Work out the finished part from the listing and answer in its coordinate system (mm). A direction names the side the tool comes from. Give positions to 0.01 mm unless a question says otherwise; leave off trailing zeros. Order: outer loops, then holes, each group sorted by start corner. A loop starts at its lowest first (then second) coordinate and runs counter-clockwise, first axis right, second up.
```python
from build123d import *

# Parameters (mm, degrees)
F1_DEPTH  = 150
F3_DEPTH  = 15
F3_FACE_R = 12.5031074182
F4_DEPTH  = 15
F4_TAPER  = -45


with BuildPart() as f1:
    # F0 (on Top) → F1 (new body)
    with BuildSketch(Plane.XY):
        Polygon((15.4211589057, 1.0175080366), (3.7976925262, 14.9808209413), (-13.0740558457, 8.2411484845), (-11.8779034096, -9.8875110716), (5.7331078234, -14.3519663908), align=None)
    extrude(amount=F1_DEPTH)

    # F2 (on face) → F3 (join)
    with BuildSketch(Plane.XY.offset(150)):
        with BuildLine():
            ThreePointArc((10.5771332585, -6.6672293454), (12.0119675412, -3.4699179964), (12.5031074182, 0))
            ThreePointArc((12.5031074182, 0), (11.7574524907, 4.2532347737), (9.6094258021, 7.9991643854))
            ThreePointArc((9.6094258021, 7.9991643854), (3.07239751, 12.119738803), (-4.6381823272, 11.6109844463))
            ThreePointArc((-4.6381823272, 11.6109844463), (-10.5771335272, 6.667228919), (-12.4759796348, -0.8231811852))
            ThreePointArc((-12.4759796348, -0.8231811852), (-9.6094258213, -7.9991643624), (-3.0723980071, -12.119738677))
            ThreePointArc((-3.0723980071, -12.119738677), (4.6381814649, -11.6109847907), (10.5771332585, -6.6672293454))
        make_face()
    extrude(amount=F3_DEPTH)

    # F3_face (on face) → F4 (join)
    with BuildSketch(Plane.XY.offset(165)):
        Circle(F3_FACE_R)
    extrude(amount=F4_DEPTH, taper=F4_TAPER)


solid = f1.part
```
1. The part is cut by section B-B (x = 0). Write down the section's boundary in (y, z).
Findings below:
outline: (-27.5, 180) - (-12.5, 165) - (-12.5, 150) - (-12.9, 150) - (-12.9, 0) - (13.46, 0) - (13.46, 150) - (12.5, 150) - (12.5, 165) - (27.5, 180) - close
2. The part is cut by section A-A (z = 60). Write down the section's boundary in (x, y).
Findings below:
outline: (-13.07, 8.24) - (-11.88, -9.89) - (5.73, -14.35) - (15.42, 1.02) - (3.8, 14.98) - close
3. Straight lines are drawn through the part: probe 1 along Z at (x, y) = (-12.5, 3); probe 2 along Z at (x, y) = (-18.5, 3); probe 3 along X at (y, z) = (3, 145). For each, find the intervals that lie inside material, in ascending order.
Findings below:
probe 1: z = 0 to 150, 165.35 to 180
probe 2: z = 171.24 to 180
probe 3: x = -12.73 to 13.77
4. Given P1, Ø5, axis at y = -9.5, z = 149.5, coming from the -X side; P2, Ø3, axis at x = -6.5, z = 91, coming from the +Y side; P3, Ø1.5, axis at x = 15.5, z = 50, coming from the +Y side, each flat-ended and moving along its own axis, determine where each tip first touches the part or whether it passes through.
Findings below:
P1: stops at x = -12.07
P2: stops at y = 11.47
P3: stops at y = 1.82
5. The mould has two halves that part along Z. Classify faces 4 (the face through (-11, 7, 150)), 5 (the face through (1, 1, 0)), 6 (the face through (-12.484, -0.696, 73.95)), 7 (the face through (0, 0, 180)): pulls with the +Z half, pulls with the -Z half, needs draft (parallel to the pull), parting line crosses it, or undercut.
Findings below:
face 4: undercut
face 5: pulls with the -Z half
face 6: needs draft
face 7: pulls with the +Z half
6. Which of the six approach directions +Z, -Z, +X, -X, +Y, -Y give full straight-line access (tool end or side, diameter ignored) to faces 1 (the face through (-4.52, 11.66, 73.95)), 2 (the face through (10.51, -6.77, 73.95)), 3 (the face through (-3.196, -12.088, 73.95))?
Findings below:
face 1: -Z, -X, +Y
face 2: -Z, +X, -Y
face 3: -Z, -X, -Y
